Autodesk Inventor part; units mm, degrees
ref_plane "XZ Plane" through (0, 0, 0) normal (0, 1, 0) x (-1, 0, 0)
ref_plane "XY Plane" through (0, 0, 0) normal (0, 0, 1) x (1, 0, 0)
sketch "Эскиз1" plane through (0, 0, 0) normal (0, 0, 1) x (1, 0, 0)
  line L0 (-120, 145) -> (120, 145)
  line L1 (120, 145) -> (120, -145)
  line L2 (120, -145) -> (-120, -145)
  line L3 (-120, -145) -> (-120, 145)
  line L4 (-120, 145) -> (120, -145) construction
  line L5 (120, 145) -> (-120, -145) construction
  point P0 (0, 0)
  dimension "d0" = 240
  dimension "d1" = 290
extrude "Выдавливание1" add sketch "Эскиз1" along normal blind 3
sketch "Эскиз2" plane through (0, 0, 3) normal (0, 0, 1) x (1, 0, 0)
  line L0 (-5, 120) -> (5, 120)
  line L1 (120, 145) -> (-120, 145)
  line L2 (0, 203) -> (0, -203)
  line L3 (-101.423, -64.3301) -> (-106.423, -55.6699)
  line L4 (106.423, -55.6699) -> (101.423, -64.3301)
  point P0 (0, 0)
  point P1 (0, 120)
  point P2 (0, 0)
  point P3 (-103.923, -60)
  point P4 (103.923, -60)
  dimension "d4" = 25
  dimension "d5" = 10
  dimension "d8" = 360
  dimension "d10" = 120
sketch "Эскиз3" plane through (0, 0, 0) normal (0, 0, -1) x (-1, 0, 0)
  circle A0 centre (17.5, 8) radius 2
  circle A1 centre (-17.5, 8) radius 2
  circle A2 centre (-100.892, -58.25) radius 1.5
  circle A3 centre (-62.7868, -36.25) radius 1.5
  circle A4 centre (100.892, -58.25) radius 1.5
  circle A5 centre (62.7868, -36.25) radius 1.5
  circle A6 centre (0, 116.5) radius 1.5
  circle A7 centre (0, 72.5) radius 1.5
  circle A8 centre (0, 0) radius 4.6
  circle A9 centre (0, 0) radius 4.65
  point P0 (0, 0)
  dimension "d13" = 0.05
extrude "Выдавливание2" cut sketch "Эскиз3" against normal through all contours A0 | A1 | A2 | A3 | A4 | A6 | A7 | A8 | A9
properties part number "верхняя пластина"
CAD build for the part. Positions are in the model's coordinates, mm. Coordinates: 2 decimals unless noted, no trailing zeros. Loops run counter-clockwise (first coordinate to the right, second up) from the corner with the lowest first, then second, coordinate; pieces in that order, holes last. Notation, with made-up numbers: (48.25, 1) - (98.25, 1) arc R30 ccw to (98.25, 23) - close; hole circle Ø6 at (80.25, -4.5). An arc over 180 degrees is marked (long way). Write item = value, one per line. Start each with the question number.
Q1. Drill centre lines: L1, parallel to X at y = -0.5, z = 1.35; L2, parallel to X at y = 116.5, z = 0.6. Where is each one in solid material? Low to high.
Q2. Pull direction X, two halves, no side cores. Call faces 1 (the cylindrical face through (-2.5, 3.92, 1.48)), 2 (the flat face through (-28, 2, 3)): pulls with the +X half, pulls with the -X half, needs draft (parallel to the pull), parting line crosses it, or undercut.
Q3. Cut at A-A, the plane y = 0. List the corners of the cut face in (x, z), then the cut area to 3 significant figures.
Q4. Flat gauge pin, fed straight in: pin 1 Ø4.5 at (x, y) = (-17.5, 8) entering from +Z. Where does the tip first touch, or does it go through?
Computed:
q1.L1 = -120 to -4.62, 4.62 to 120
q1.L2 = -120 to -1.5, 1.5 to 120
q2.face_1 = undercut
q2.face_2 = needs draft
q3.outline = (-120, 0) - (-4.65, 0) - (-4.65, 3) - (-120, 3) - close; (4.65, 0) - (120, 0) - (120, 3) - (4.65, 3) - close
q3.area = 692 mm²
q4.pin_1 = 3
